Part model, mm, in its own coordinate system. Face numbers are marked on the shaded views. A direction names the side the tool comes from. Round coordinates to 2 decimals unless told otherwise and drop trailing zeros. Order: outer loops, then holes, each group sorted by start corner. A loop starts at its lowest first (then second) coordinate and runs counter-clockwise, first axis right, second up. Notation, with made-up numbers: (-36, 51) - (-23, 51) arc R15 cw to (-23, 72) - close; hole circle Ø1 at (64.5, 42). An arc over 180 degrees is marked (long way). Return JSON: item names as keys, results as strings. Group by question number.
Item 1: Drop flat-ended pins along their axis: pin 1 (1.5 mm diameter, centred on y = 13, z = 35, fed in from +X); pin 2 (2 mm diameter, centred on x = -29, z = 31, fed in from +Y); pin 3 (4 mm diameter, centred on x = 30.5, z = 7, fed in from +Y). Give the stop position or say it passes through.
Item 2: Saw through at B-B on y = 7.5. List the corners of the cut face in (x, z), and give its area (3 significant figures).
Item 3: Saw through at A-A on x = 0. List the corners of the cut face in (y, z), and give its area (3 significant figures).
Item 4: Saw through at C-C on y = 50. List the corners of the cut face in (x, z).
Item 5: Two-plate mould, pull along X, no slides. Class the marked faces 3, 4 and 5: released by +X, released by -X, zero draft, split by the parting line, or undercut.
Item 6: Probe probe 1 along X at (y, z) = (-10, 0); probe 2 along Y at (x, z) = (-3, 0). List the from-to ranges inside material, lowest first.
Item 7: Tool access for the marked faces 1 and 2: list every direction of +Z, -Z, +X, -X, +Y, -Y with a clear straight run to the whole face (end or side of a thin tool).
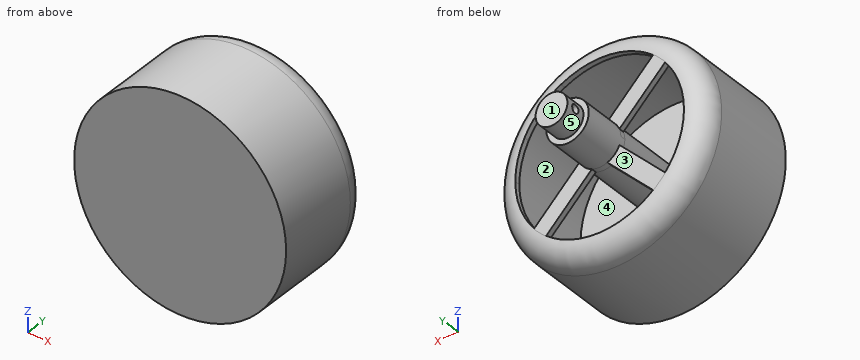
```python
from build123d import *
from build123d.topology import SkipClean

# Parameters (mm, degrees)
SKETCH2_R               = 10
BOSS_EXTRUDE1_DEPTH     = 30
CUT_EXTRUDE1_START      = -10
SKETCH3_R               = 10
SKETCH3_R_2             = 7.5
CUT_EXTRUDE1_DEPTH      = 10
CUT_EXTRUDE3_DEPTH      = 10
CUT_EXTRUDE3_DEPTH_BACK = 10
SKETCH5_R               = 2
CUT_EXTRUDE4_START      = -10
CUT_EXTRUDE4_DEPTH      = 10
FILLET2_R               = 10
BOSS_EXTRUDE2_START     = -67.5
SKETCH7_R               = 10
BOSS_EXTRUDE2_DEPTH     = 67.5


with BuildPart() as part:
    # Sketch1 → Revolve1 (revolve)
    with BuildSketch(Plane.XY):
        Polygon((50, 25), (0, 25), (0, 22.5), (45, 22.5), (45, -22.5), (0, -22.5), (0, -25), (50, -25), align=None)
    revolve(axis=Axis((0, -25, 0), (0, 1, 0)))

    # Sketch2 → Boss-Extrude1 (add)
    with BuildSketch(Plane(origin=(0, 25, 0), x_dir=(1, 0, 0), z_dir=(0, 1, 0))):
        with Locations(Location((0, 0, 0), (0, 0, 180))):
            Circle(SKETCH2_R)
    extrude(amount=BOSS_EXTRUDE1_DEPTH)

    # Sketch3 → Cut-Extrude1 (cut)
    with BuildSketch(Plane(origin=(0, 55, 0), x_dir=(1, 0, 0), z_dir=(0, 1, 0)).offset(CUT_EXTRUDE1_START)):
        with Locations(Location((0, 0, 0), (0, 0, 180))):
            Circle(SKETCH3_R)
        with Locations(Location((0, 0, 0), (0, 0, 180))):
            Circle(SKETCH3_R_2, mode=Mode.SUBTRACT)
    extrude(amount=CUT_EXTRUDE1_DEPTH, mode=Mode.SUBTRACT)

    # Sketch5 → Cut-Extrude3 (cut, two sides: drawn at the far end of the back side and taken through both)
    with BuildSketch(Plane(origin=(0, 0, 0), x_dir=(0, 0, -1), z_dir=(1, 0, 0)).offset(-CUT_EXTRUDE3_DEPTH_BACK)):
        with Locations(Location((0, 50, 0), (0, 0, 180))):
            Circle(SKETCH5_R)
    extrude(amount=CUT_EXTRUDE3_DEPTH + CUT_EXTRUDE3_DEPTH_BACK, mode=Mode.SUBTRACT)

    # Sketch6 → Cut-Extrude4 (cut)
    with SkipClean():  # the faces are left unmerged after this step: merging them gives an invalid solid
        with BuildSketch(Plane(origin=(0, 25, 0), x_dir=(1, 0, 0), z_dir=(0, 1, 0)).offset(CUT_EXTRUDE4_START)):
            with BuildLine():
                ThreePointArc((18.327704801, 35.312767957), (0, 39.785629869), (-18.327704801, 35.312767957))
                Line((-18.327704801, 35.312767957), (18.327704801, 35.312767957))
            make_face()
            with BuildLine():
                Line((-25.198784951, 30.788270186), (-3.663513289, 9.304766004))
                ThreePointArc((-3.663513289, 9.304766004), (0, 10), (3.663513289, 9.304766004))
                Line((3.663513289, 9.304766004), (25.198784951, 30.788270186))
                ThreePointArc((25.198784951, 30.788270186), (21.880507251, 33.228598323), (18.327704801, 35.312767957))
                Line((18.327704801, 35.312767957), (-18.327704801, 35.312767957))
                ThreePointArc((-18.327704801, 35.312767957), (-21.880507251, 33.228598323), (-25.198784951, 30.788270186))
            make_face()
            with BuildLine():
                Line((30.848827824, 25.124612751), (9.313556162, 3.641108569))
                ThreePointArc((9.313556162, 3.641108569), (9.826890699, 1.852624946), (10, 0))
                ThreePointArc((10, 0), (9.826890699, -1.852624946), (9.313556162, -3.641108569))
                Line((9.313556162, -3.641108569), (30.848827824, -25.124612751))
                ThreePointArc((30.848827824, -25.124612751), (33.305743158, -21.762900008), (35.397858964, -18.162817094))
                Line((35.397858964, -18.162817094), (35.397858964, 18.162817094))
                ThreePointArc((35.397858964, 18.162817094), (33.305743158, 21.762900008), (30.848827824, 25.124612751))
            make_face()
            with BuildLine():
                ThreePointArc((39.785629869, 0), (38.673133173, 9.342650297), (35.397858964, 18.162817094))
                Line((35.397858964, 18.162817094), (35.397858964, -18.162817094))
                ThreePointArc((35.397858964, -18.162817094), (38.673133173, -9.342650297), (39.785629869, 0))
            make_face()
            with BuildLine():
                ThreePointArc((3.663513289, -9.304766004), (0, -10), (-3.663513289, -9.304766004))
                Line((-3.663513289, -9.304766004), (-25.198784951, -30.788270186))
                ThreePointArc((-25.198784951, -30.788270186), (-21.880507251, -33.228598323), (-18.327704801, -35.312767957))
                Line((-18.327704801, -35.312767957), (18.327704801, -35.312767957))
                ThreePointArc((18.327704801, -35.312767957), (21.880507251, -33.228598323), (25.198784951, -30.788270186))
                Line((25.198784951, -30.788270186), (3.663513289, -9.304766004))
            make_face()
            with BuildLine():
                Line((18.327704801, -35.312767957), (-18.327704801, -35.312767957))
                ThreePointArc((-18.327704801, -35.312767957), (0, -39.785629869), (18.327704801, -35.312767957))
            make_face()
            with BuildLine():
                ThreePointArc((-9.313556162, -3.641108569), (-10, 0), (-9.313556162, 3.641108569))
                Line((-9.313556162, 3.641108569), (-30.848827824, 25.124612751))
                ThreePointArc((-30.848827824, 25.124612751), (-33.305743158, 21.762900008), (-35.397858964, 18.162817094))
                Line((-35.397858964, 18.162817094), (-35.397858964, -18.162817094))
                ThreePointArc((-35.397858964, -18.162817094), (-33.305743158, -21.762900008), (-30.848827824, -25.124612751))
                Line((-30.848827824, -25.124612751), (-9.313556162, -3.641108569))
            make_face()
            with BuildLine():
                Line((-35.397858964, -18.162817094), (-35.397858964, 18.162817094))
                ThreePointArc((-35.397858964, 18.162817094), (-39.785629869, 0), (-35.397858964, -18.162817094))
            make_face()
        extrude(amount=CUT_EXTRUDE4_DEPTH, mode=Mode.SUBTRACT)

    # Fillet2
    fillet2_edges = [part.edges().sort_by_distance(p)[0] for p in [
        (-50, 25, 0),
    ]]
    fillet(fillet2_edges, radius=FILLET2_R)

    # Sketch7 → Boss-Extrude2 (add)
    with SkipClean():  # the faces are left unmerged after this step: merging them gives an invalid solid
        with BuildSketch(Plane(origin=(0, 45, 0), x_dir=(1, 0, 0), z_dir=(0, 1, 0)).offset(BOSS_EXTRUDE2_START)):
            with Locations(Location((0, 0, 0), (0, 0, 180))):
                Circle(SKETCH7_R)
        extrude(amount=BOSS_EXTRUDE2_DEPTH)


solid = part.part
```
Filled in:
{
 "1": {"pin 1": "stops at x = 36.43", "pin 2": "stops at y = 24.89", "pin 3": "stops at y = -22.5"},
 "2": {"outline": "circle Ø100 at (0, 0); circle Ø20 at (0, 0); hole circle Ø90 at (0, 0)", "area": "1,810 mm^2"},
 "3": {"outline": "(-25, -50) - (15, -50) arc R10 ccw to (25, -40) - (25, -39.79) - (22.5, -39.79) - (22.5, -45) - (-22.5, -45) - (-22.5, -10) - (45, -10) - (45, -7.5) - (55, -7.5) - (55, 7.5) - (45, 7.5) - (45, 10) - (-22.5, 10) - (-22.5, 45) - (22.5, 45) - (22.5, 39.79) - (25, 39.79) - (25, 40) arc R10 ccw to (15, 50) - (-25, 50) - close; hole circle Ø4 at (50, 0)", "area": "2,200 mm^2"},
 "4": {"outline": "(-7.23, -2) arc R7.5 ccw to (7.23, -2) - close; (-7.23, 2) - (7.23, 2) arc R7.5 ccw to start"},
 "5": {"face 3": "zero draft", "face 4": "undercut", "face 5": "split by the parting line"},
 "6": {"probe 1": "x = -50 to -45, -10 to 10, 45 to 50", "probe 2": "y = -25 to 48, 52 to 55"},
 "7": {"face 1": "+Z, -Z, +X, -X, +Y", "face 2": "none"}
}
